from build123d import *

# Parameters (mm, degrees)
SKETCH1_W           = 28
SKETCH1_H           = 48
BOSS_EXTRUDE1_DEPTH = 23
SKETCH3_W           = 24
SKETCH3_H           = 44
CUT_EXTRUDE1_DEPTH  = 19.5
SKETCH4_W           = 7
SKETCH4_H           = 8
BOSS_EXTRUDE2_DEPTH = 3.5
SKETCH5_R           = 1.7
CUT_EXTRUDE5_DEPTH  = 3.5
CUT_EXTRUDE7_DEPTH  = 50


with BuildPart() as part:
    # Sketch1 → Boss-Extrude1 (new body)
    with BuildSketch(Plane(origin=(0, 0, 0), x_dir=(1, 0, 0), z_dir=(0, 1, 0))):
        Rectangle(SKETCH1_W, SKETCH1_H)
    extrude(amount=BOSS_EXTRUDE1_DEPTH)

    # Sketch3 → Cut-Extrude1 (cut)
    with BuildSketch(Plane(origin=(0, 23, 0), x_dir=(1, 0, 0), z_dir=(0, 1, 0))):
        Rectangle(SKETCH3_W, SKETCH3_H)
    extrude(amount=-CUT_EXTRUDE1_DEPTH, mode=Mode.SUBTRACT)

    # Sketch4 → Boss-Extrude2 (add)
    with BuildSketch(Plane.XZ):
        with Locations((17.5, 17.395203427)):
            Rectangle(SKETCH4_W, SKETCH4_H)
        with Locations((17.5, -17.574178575)):
            Rectangle(SKETCH4_W, SKETCH4_H)
        with Locations((-17.5, -17.574178575)):
            Rectangle(SKETCH4_W, SKETCH4_H)
        with Locations((-17.5, 17.395203427)):
            Rectangle(SKETCH4_W, SKETCH4_H)
    extrude(amount=-BOSS_EXTRUDE2_DEPTH)

    # Sketch5 → Cut-Extrude5 (cut)
    with BuildSketch(Plane.XZ):
        with Locations(Location((-17.5, 17.395203427, 0), (0, 0, 270))):
            Circle(SKETCH5_R)
        with Locations(Location((-17.5, -17.574178575, 0), (0, 0, 270))):
            Circle(SKETCH5_R)
        with Locations(Location((17.5, -17.574178575, 0), (0, 0, 270))):
            Circle(SKETCH5_R)
        with Locations(Location((17.5, 17.395203427, 0), (0, 0, 270))):
            Circle(SKETCH5_R)
    extrude(amount=-CUT_EXTRUDE5_DEPTH, mode=Mode.SUBTRACT)

    # Sketch7 → Cut-Extrude7 (cut)
    with BuildSketch(Plane.XY.offset(24)):
        with BuildLine():
            Line((3, 25.962103345), (3, 8.556782005))
            ThreePointArc((3, 8.556782005), (0, 5.556782005), (-3, 8.556782005))
            Line((-3, 8.556782005), (-3, 25.962103345))
            ThreePointArc((-3, 25.962103345), (0, 28.962103345), (3, 25.962103345))
        make_face()
    extrude(amount=-CUT_EXTRUDE7_DEPTH, mode=Mode.SUBTRACT)


solid = part.part
Here's how the part is built. I have some questions about the finished solid (model axes, mm). A direction names the side the tool comes from. Give positions to 0.01 mm unless a question says otherwise; leave off trailing zeros. Order: outer loops, then holes, each group sorted by start corner. A loop starts at its lowest first (then second) coordinate and runs counter-clockwise, first axis right, second up. Notation, with made-up numbers: M 66.5,18.5 L 115.5,18.5 A24 cw 115.5,40.5 Z; hole C 73.5,35.5 d9. An arc over 180 degrees is marked long. Answer as a JSON object with one key per item and string values. Group by question number.
1) On a 3-axis mill with a long thin cutter (end or side, diameter ignored), from which of +Z, -Z, +X, -X, +Y, -Y can I reach the whole of each face in a straight line? I mean faces 4 (the flat face through (-17.5, 3.5, -15.7)), 5 (the flat face through (-18, 2, 21.395)), 6 (the flat face through (-3, 16, 23)). Say none if no direction works.
2) I'm going to push flat-ended pins straight in: pin 1 Ø2 at (y, z) = (8.5, 16) entering from +X; pin 2 Ø3 at (x, y) = (18, 1) entering from -Z; pin 3 Ø11.5 at (y, z) = (15, -10.5) entering from -X; pin 4 Ø1 at (x, y) = (-16, 8) entering from -Z. Where does each tip first touch, or does it pass through?
3) Suppose I cut it at D-D, the plane z = -18. Write out the boundary of the cut face in (x, y), plus the area to 3 significant figures.
4) Please list where these lines run through material, in increasing order: L1, parallel to X at y = 11.5, z = -4.5; L2, parallel to Z at x = 9.5, y = 8.5; L3, parallel to Y at x = -11, z = 7.5. Write a range as [from, to].
5) We'd pull the mould along Z, two halves only. Please class faces 1 (the flat face through (17, 2, 21.395)), 2 (the flat face through (17, 2, 13.395)), 3 (the flat face through (13, 23, 5)): pulls with the +Z half, pulls with the -Z half, needs draft (parallel to the pull), parting line crosses it, or undercut.
6) Suppose I cut it at A-A, the plane x = 17.5. Write out the boundary of the cut face in (y, z).
7) Suppose I cut it at C-C, the plane z = -2.5. Write out the boundary of the cut face in (x, y).
8) Suppose I cut it at B-B, the plane y = 10. Write out the boundary of the cut face in (x, z).
Results found:
{
 "1": {"face 4": "+Z, -Z, -X, +Y", "face 5": "+Z, -X, +Y, -Y", "face 6": "+Z, -Z, +Y"},
 "2": {"pin 1": "x = 14", "pin 2": "z = -21.57", "pin 3": "x = -14", "pin 4": "through"},
 "3": {"outline": "M -21,0 L -19.15,0 L -19.15,3.5 L -21,3.5 Z; M -15.85,0 L 15.85,0 L 15.85,3.5 L 14,3.5 L 14,23 L 12,23 L 12,3.5 L -12,3.5 L -12,23 L -14,23 L -14,3.5 L -15.85,3.5 Z; M 19.15,0 L 21,0 L 21,3.5 L 19.15,3.5 Z", "area": "202 mm²"},
 "4": {"L1": "[-14, -12], [12, 14]", "L2": "[-24, -22], [22, 24]", "L3": "[0, 3.5]"},
 "5": {"face 1": "pulls with the +Z half", "face 2": "undercut", "face 3": "needs draft"},
 "6": {"outline": "M 0,-21.57 L 3.5,-21.57 L 3.5,-19.27 L 0,-19.27 Z; M 0,-15.87 L 3.5,-15.87 L 3.5,-13.57 L 0,-13.57 Z; M 0,13.4 L 3.5,13.4 L 3.5,15.7 L 0,15.7 Z; M 0,19.1 L 3.5,19.1 L 3.5,21.4 L 0,21.4 Z"},
 "7": {"outline": "M -14,0 L 14,0 L 14,23 L 12,23 L 12,3.5 L -12,3.5 L -12,23 L -14,23 Z"},
 "8": {"outline": "M -14,-24 L -3,-24 L -3,-22 L -12,-22 L -12,22 L -3,22 L -3,24 L -14,24 Z; M 3,-24 L 14,-24 L 14,24 L 3,24 L 3,22 L 12,22 L 12,-22 L 3,-22 Z"}
}
